Design review of the part built by this model. Coordinates are the model's own, in mm. Round coordinates to 2 decimals unless told otherwise and drop trailing zeros. Write each loop counter-clockwise with the first axis right and the second up, starting at its lowest first coordinate (ties: lowest second). Pieces come first, ordered by that corner, then holes. Notation, with made-up numbers: (-1.75, 83) -> (31.25, 83) arc R27 ccw to (31.25, 118) -> close; hole circle Ø1 at (29, 6.5). An arc over 180 degrees is marked (long way). Write item = value, one per line. Start each with the question number.
Item 1: To check wall thickness, follow L1, parallel to X at y = 2.9, z = 48.2; L2, parallel to X at y = 3.85, z = 35.7; L3, parallel to X at y = 3.9, z = -53.2. State the ranges of each line that lie inside material, in increasing order.
Item 2: Add section D-D, the plane z = 23.2. State the section outline as (x, y) points.
Item 3: Add section C-C, the plane z = -28.5. State the section outline as (x, y) points.
Item 4: Add section A-A, the plane x = -48.05. State the section outline as (y, z) points, then the cut area to 3 significant figures.
Item 5: Add section B-B, the plane z = 48.2. State the section outline as (x, y) points.
Item 6: For pin 1 Ø1.9 at (x, z) = (48.05, 48.2) entering from +Y; pin 2 Ø1.5 at (x, y) = (60, 1.5) entering from -Z; pin 3 Ø2.5 at (x, y) = (-59, 1.5) entering from -Z; pin 4 Ø2.5 at (x, y) = (60, 3.5) entering from -Z, all flat-tipped, find the tip position at first contact; note any pin that passes through.
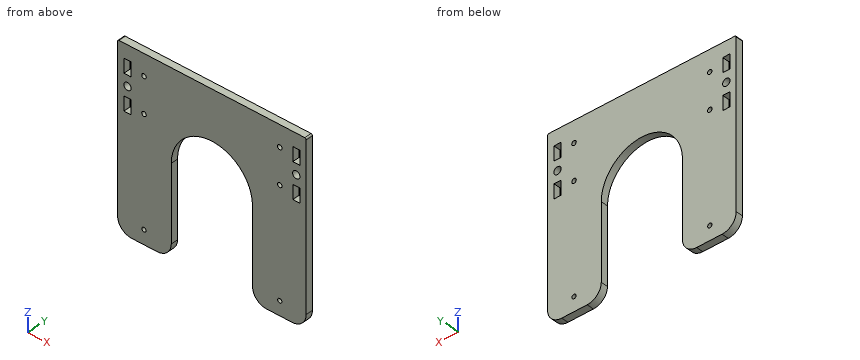
from build123d import *

# Parameters (mm, degrees)
SKETCH1_W           = 133.5
SKETCH1_H           = 126.4
SKETCH1_R           = 2.6
SKETCH1_R_2         = 1.6
SKETCH1_W_2         = 5
SKETCH1_H_2         = 10
BOSS_EXTRUDE1_DEPTH = 5
CUT_EXTRUDE2_DEPTH  = 10
FILLET2_R           = 10
CUT_EXTRUDE3_REACH  = 94.059
SKETCH5_R           = 1.6
SKETCH5_R_2         = 1.5
FILLET3_R           = 1


with BuildPart() as part:
    # Sketch1 → Boss-Extrude1 (new body)
    with BuildSketch(Plane(origin=(0, 0, 0), x_dir=(1, 0, 0), z_dir=(0, 1, 0))):
        Rectangle(SKETCH1_W, SKETCH1_H)
        with Locations(Location((-59.75, -35.7, 0), (0, 0, 270))):
            Circle(SKETCH1_R, mode=Mode.SUBTRACT)
        with Locations(Location((59.75, -35.7, 0), (0, 0, 90))):
            Circle(SKETCH1_R, mode=Mode.SUBTRACT)
        with Locations(Location((-48.05, -48.2, 0), (0, 0, 270))):
            Circle(SKETCH1_R_2, mode=Mode.SUBTRACT)
        with Locations(Location((48.05, -48.2, 0), (0, 0, 90))):
            Circle(SKETCH1_R_2, mode=Mode.SUBTRACT)
        with Locations((-59.75, -48.2)):
            Rectangle(SKETCH1_W_2, SKETCH1_H_2, mode=Mode.SUBTRACT)
        with Locations((-59.75, -23.2)):
            Rectangle(SKETCH1_W_2, SKETCH1_H_2, mode=Mode.SUBTRACT)
        with Locations((59.75, -23.2)):
            Rectangle(SKETCH1_W_2, SKETCH1_H_2, mode=Mode.SUBTRACT)
        with Locations((59.75, -48.2)):
            Rectangle(SKETCH1_W_2, SKETCH1_H_2, mode=Mode.SUBTRACT)
    extrude(amount=BOSS_EXTRUDE1_DEPTH)

    # Sketch2 → Cut-Extrude2 (cut)
    with BuildSketch(Plane(origin=(0, 5, 0), x_dir=(1, 0, 0), z_dir=(0, 1, 0))):
        with BuildLine():
            Line((-28.75, 86.678700037), (-28.75, 0))
            ThreePointArc((-28.75, 0), (0, -28.75), (28.75, 0))
            Line((28.75, 0), (28.75, 86.678700037))
            Line((28.75, 86.678700037), (-28.75, 86.678700037))
        make_face()
    extrude(amount=-CUT_EXTRUDE2_DEPTH, mode=Mode.SUBTRACT)

    # Fillet2
    fillet2_edges = [part.edges().sort_by_distance(p)[0] for p in [
        (-66.75, 2.5, -63.2),
        (66.75, 2.5, -63.2),
        (-28.75, 2.5, -63.2),
        (28.75, 2.5, -63.2),
    ]]
    fillet(fillet2_edges, radius=FILLET2_R)

    # Sketch5 → Cut-Extrude3 (cut, up to next)
    with BuildSketch(Plane.XZ, mode=Mode.PRIVATE) as cut_extrude3_sk1:
        with Locations(Location((48.05, 23.2, 0), (0, 0, 270))):
            Circle(SKETCH5_R)
    cut_extrude3_tool1 = extrude(cut_extrude3_sk1.sketch, amount=-CUT_EXTRUDE3_REACH, mode=Mode.PRIVATE) & part.part
    # Sketch5 → Cut-Extrude3 (cut, up to next)
    with BuildSketch(Plane.XZ, mode=Mode.PRIVATE) as cut_extrude3_sk2:
        with Locations(Location((48.05, -53.2, 0), (0, 0, 270))):
            Circle(SKETCH5_R_2)
    cut_extrude3_tool2 = extrude(cut_extrude3_sk2.sketch, amount=-CUT_EXTRUDE3_REACH, mode=Mode.PRIVATE) & part.part
    # Sketch5 → Cut-Extrude3 (cut, up to next)
    with BuildSketch(Plane.XZ, mode=Mode.PRIVATE) as cut_extrude3_sk3:
        with Locations(Location((-48.05, -53.2, 0), (0, 0, 90))):
            Circle(SKETCH5_R_2)
    cut_extrude3_tool3 = extrude(cut_extrude3_sk3.sketch, amount=-CUT_EXTRUDE3_REACH, mode=Mode.PRIVATE) & part.part
    # Sketch5 → Cut-Extrude3 (cut, up to next)
    with BuildSketch(Plane.XZ, mode=Mode.PRIVATE) as cut_extrude3_sk4:
        with Locations(Location((-48.05, 23.2, 0), (0, 0, 90))):
            Circle(SKETCH5_R)
    cut_extrude3_tool4 = extrude(cut_extrude3_sk4.sketch, amount=-CUT_EXTRUDE3_REACH, mode=Mode.PRIVATE) & part.part
    add(cut_extrude3_tool1.solids().sort_by_distance((48.05, 0, 23.2))[0], mode=Mode.SUBTRACT)
    add(cut_extrude3_tool2.solids().sort_by_distance((48.05, 0, -53.2))[0], mode=Mode.SUBTRACT)
    add(cut_extrude3_tool3.solids().sort_by_distance((-48.05, 0, -53.2))[0], mode=Mode.SUBTRACT)
    add(cut_extrude3_tool4.solids().sort_by_distance((-48.05, 0, 23.2))[0], mode=Mode.SUBTRACT)

    # Fillet3
    fillet3_edges = [part.edges().sort_by_distance(p)[0] for p in [
        (66.75, 2.5, 63.2),
        (-66.75, 2.5, 63.2),
    ]]
    fillet(fillet3_edges, radius=FILLET3_R)


solid = part.part
Result set:
q1.L1 = -66.75 to -62.25, -57.25 to -49.65, -46.45 to 46.45, 49.65 to 57.25, 62.25 to 66.75
q1.L2 = -66.75 to -62.35, -57.15 to 57.15, 62.35 to 66.75
q1.L3 = -66.75 to -49.55, -46.55 to -28.75, 28.75 to 46.55, 49.55 to 66.75
q2.outline = (-66.75, 0) -> (-62.25, 0) -> (-62.25, 5) -> (-66.75, 5) -> close; (-57.25, 0) -> (-49.65, 0) -> (-49.65, 5) -> (-57.25, 5) -> close; (-46.45, 0) -> (-16.98, 0) -> (-16.98, 5) -> (-46.45, 5) -> close; (16.98, 0) -> (46.45, 0) -> (46.45, 5) -> (16.98, 5) -> close; (49.65, 0) -> (57.25, 0) -> (57.25, 5) -> (49.65, 5) -> close; (62.25, 0) -> (66.75, 0) -> (66.75, 5) -> (62.25, 5) -> close
q3.outline = (-66.75, 0) -> (-28.75, 0) -> (-28.75, 5) -> (-66.75, 5) -> close; (28.75, 0) -> (66.75, 0) -> (66.75, 5) -> (28.75, 5) -> close
q4.outline = (0, -63.2) -> (5, -63.2) -> (5, -54.7) -> (0, -54.7) -> close; (0, -51.7) -> (5, -51.7) -> (5, 21.6) -> (0, 21.6) -> close; (0, 24.8) -> (5, 24.8) -> (5, 46.6) -> (0, 46.6) -> close; (0, 49.8) -> (5, 49.8) -> (5, 63.2) -> (0, 63.2) -> close
q4.area = 585 mm²
q5.outline = (-66.75, 0) -> (-62.25, 0) -> (-62.25, 5) -> (-66.75, 5) -> close; (-57.25, 0) -> (-49.65, 0) -> (-49.65, 5) -> (-57.25, 5) -> close; (-46.45, 0) -> (46.45, 0) -> (46.45, 5) -> (-46.45, 5) -> close; (49.65, 0) -> (57.25, 0) -> (57.25, 5) -> (49.65, 5) -> close; (62.25, 0) -> (66.75, 0) -> (66.75, 5) -> (62.25, 5) -> close
q6.pin_1 = through
q6.pin_2 = -62.88
q6.pin_3 = -63.15
q6.pin_4 = -63
